The model under review builds one solid part; all positions refer to its coordinate system, in mm. Face numbers are marked on the shaded views. A direction names the side the tool comes from. Coordinates: 2 decimals unless noted, no trailing zeros. Loops run counter-clockwise (first coordinate to the right, second up) from the corner with the lowest first, then second, coordinate; pieces in that order, holes last. Notation, with made-up numbers: (75.5, -34.5) - (104.5, -34.5) arc R21 cw to (104.5, -8.5) - close; hole circle Ø9 at (24, 15.5). An arc over 180 degrees is marked (long way). One line per item, written item: value. Start each with the question number.
1. We need section B-B, the plane z = -3.75. Give the boundary of the cut face in (x, y).
2. We need section C-C, the plane z = -6.25. Give the boundary of the cut face in (x, y).
3. Mouldability with a two-part tool opening along X and no side actions: class the marked faces 1, 2, 3 and 4 as +X half, -X half, draft (parallel to the pull), parting line (faces both ways), or undercut.
4. To check wall thickness, follow line 1 (X direction, y = 5.5, z = -11.25); line 2 (Y direction, x = 0, z = -9.05); line 3 (Y direction, x = 0, z = -5.5). State the ranges of each line that lie inside material, in increasing order.
5. Insertion check: P1, Ø4, axis at y = 11, z = -2, coming from the -X side; P2, Ø5, axis at x = 1.5, y = 7.5, coming from the -Z side; P3, Ø2, axis at x = 31.5, y = 9.5, coming from the -Z side. Each pin has a flat end and moves straight along its axis. Give the tip position at first contact, or say it passes through.
6. We need section A-A, the plane x = 0. Give the boundary of the cut face in (y, z).
7. For the marked faces 5, 6, 7 and 8, list the 3-axis set-ups (+Z, -Z, +X, -X, +Y, -Y) from which the entire face can be reached by the end or side of a thin tool; tool diameter is ignored.
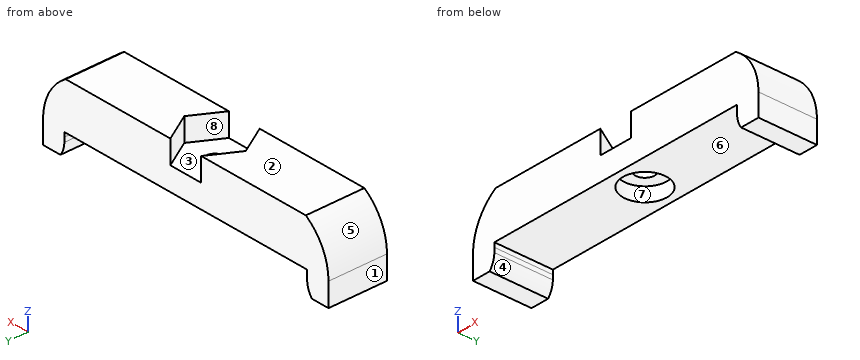
from build123d import *

# Parameters (mm, degrees)
EXTRUDE_1_DEPTH     = 12.65
CUT_EXTRUDE_1_DEPTH = 5
SKETCH_3_R          = 4.75
CUT_EXTRUDE_2_DEPTH = 3
SKETCH_6_R          = 2.1
CUT_EXTRUDE_5_DEPTH = 10
FILLET_3_R          = 5
FILLET_4_R          = 5
FILLET_6_R          = 1
FILLET_7_R          = 1
CUT_EXTRUDE_6_DEPTH = 15


with BuildPart() as part:
    # 草图1 → 凸台-拉伸1 (new body)
    with BuildSketch(Plane(origin=(0, 0, 0), x_dir=(1, 0, 0), z_dir=(0, 1, 0))):
        with BuildLine():
            Line((-28.6, 0), (28.6, 0))
            ThreePointArc((28.6, 0), (32.562096374, 4.25705164), (34, 9.892043165))
            Line((34, 9.892043165), (34, 17.266133288))
            Line((34, 17.266133288), (28.9, 15))
            Line((28.9, 15), (28.9, 10))
            Line((28.9, 10), (-28.9, 10))
            Line((-28.9, 10), (-28.9, 15))
            Line((-28.9, 15), (-34, 17.266133288))
            Line((-34, 17.266133288), (-34, 9.892043165))
            ThreePointArc((-34, 9.892043165), (-32.562096374, 4.25705164), (-28.6, 0))
        make_face()
    extrude(amount=EXTRUDE_1_DEPTH)

    # 草图2 → 切除-拉伸1 (cut)
    with BuildSketch(Plane.XY):
        Polygon((-7.32, 6.32), (-3.66, -0.019305956), (3.66, -0.019305956), (7.32, 6.32), (3.66, 12.659305956), (-3.66, 12.659305956), align=None)
    extrude(amount=-CUT_EXTRUDE_1_DEPTH, mode=Mode.SUBTRACT)

    # 草图3 → 切除-拉伸2 (cut)
    with BuildSketch(Plane(origin=(0, 0, -10), x_dir=(-1, 0, 0), z_dir=(0, 0, -1))):
        with Locations((0, 6.32)):
            Circle(SKETCH_3_R)
    extrude(amount=-CUT_EXTRUDE_2_DEPTH, mode=Mode.SUBTRACT)

    # 草图6 → 切除-拉伸5 (cut)
    with BuildSketch(Plane.XY.offset(-5)):
        with Locations((0, 6.32)):
            Circle(SKETCH_6_R)
    extrude(amount=-CUT_EXTRUDE_5_DEPTH, mode=Mode.SUBTRACT)

    # 圆角3
    fillet_3_edges = [part.edges().sort_by_distance(p)[0] for p in [
        (-28.9, 6.325, -15),
    ]]
    fillet(fillet_3_edges, radius=FILLET_3_R)

    # 圆角4
    fillet_4_edges = [part.edges().sort_by_distance(p)[0] for p in [
        (28.9, 6.325, -15),
    ]]
    fillet(fillet_4_edges, radius=FILLET_4_R)

    # 圆角6
    fillet_6_edges = [part.edges().sort_by_distance(p)[0] for p in [
        (34, 6.325, -17.266133288),
    ]]
    fillet(fillet_6_edges, radius=FILLET_6_R)

    # 圆角7
    fillet_7_edges = [part.edges().sort_by_distance(p)[0] for p in [
        (-34, 6.325, -17.266133288),
    ]]
    fillet(fillet_7_edges, radius=FILLET_7_R)

    # 草图7 → 切除-拉伸6 (cut)
    with BuildSketch(Plane.XZ):
        Polygon((28.903354644, -10.942236709), (27.407544443, -14.683649227), (28.903354644, -17.343343862), (36.500549605, -19.187562633), (35.643870018, -14.683649227), (31.998035106, -14.683649227), (28.903354644, -14.683649227), align=None)
        Polygon((-28.903354644, -10.942236709), (-27.711217355, -14.930549055), (-28.903354644, -15.756236567), (-29.008862033, -15.781540844), (-34.951049449, -20.851021688), (-36.720724333, -14.930549055), (-32.176496035, -14.930549055), (-28.903354644, -14.930549055), align=None)
    extrude(amount=-CUT_EXTRUDE_6_DEPTH, mode=Mode.SUBTRACT)


solid = part.part
Findings below:
1. outline: (-32.27, 0) - (-3.67, 0) - (-7.32, 6.32) - (-3.67, 12.65) - (-32.27, 12.65) - close; (3.67, 0) - (32.27, 0) - (32.27, 12.65) - (3.67, 12.65) - (7.32, 6.32) - close
2. outline: (-33.42, 0) - (33.42, 0) - (33.42, 12.65) - (-33.42, 12.65) - close; hole circle Ø4.2 at (0, 6.32)
3. face 1: -X half
3. face 2: draft
3. face 3: undercut
3. face 4: undercut
4. line 1: -34 to -28.9, 28.9 to 34
4. line 2: 0 to 1.57, 11.07 to 12.65
4. line 3: 0 to 4.22, 8.42 to 12.65
5. P1: x = -32.42
5. P2: z = -7
5. P3: z = -14.68
6. outline: (0, -10) - (1.57, -10) - (1.57, -7) - (4.22, -7) - (4.22, -5) - (0, -5) - close; (8.42, -7) - (11.07, -7) - (11.07, -10) - (12.65, -10) - (12.65, -5) - (8.42, -5) - close
7. face 5: +Z, -X, +Y, -Y
7. face 6: -Z, +Y, -Y
7. face 7: -Z
7. face 8: +Z
